Can you work these out from the model? Positions are in its coordinate system, mm. Face numbers are marked on the shaded views. A direction names the side the tool comes from. Give positions to 0.01 mm unless a question says otherwise; leave off trailing zeros. Order: outer loops, then holes, each group sorted by start corner. A loop starts at its lowest first (then second) coordinate and runs counter-clockwise, first axis right, second up. Notation, with made-up numbers: (21.5, 7.25) - (36.5, 7.25) arc R32 cw to (36.5, 41.25) - close; hole circle Ø5 at (18, 32). An arc over 180 degrees is marked (long way). Answer as CSV lines item,"result".
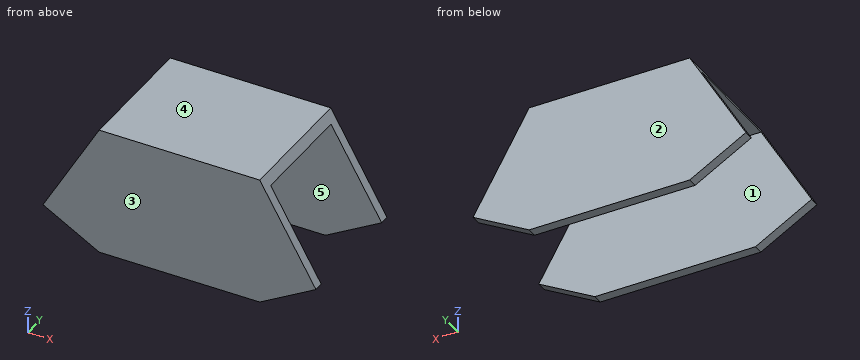
```python
from build123d import *

# Parameters (mm, degrees)
EXTRUDE_1_DEPTH = 40
SHELL_1_T       = -3


with BuildPart() as part:
    # 草图1 → 凸台-拉伸1 (new body)
    with BuildSketch(Plane(origin=(0, 0, 0), x_dir=(1, 0, 0), z_dir=(0, 1, 0))):
        Polygon((-25, -16.701458194), (25, -16.701458194), (42.5, 13.609430939), (25, 23.487817083), (-25, 23.487817083), (-42.5, 13.609430939), align=None)
    extrude(amount=EXTRUDE_1_DEPTH)

    # 抽壳1
    shell_1_openings = [part.faces().sort_by_distance(p)[0] for p in [
        (-33.75, 20, -18.548624011),
        (0, 20, -23.487817083),
        (33.75, 20, -18.548624011),
        (33.75, 20, 1.546013628),
        (-33.75, 20, 1.546013628),
    ]]
    offset(amount=SHELL_1_T, openings=shell_1_openings, kind=Kind.INTERSECTION)


solid = part.part
```
1) I want a section at C-C on x = 36.5. Write out the boundary of the cut face in (y, z).
Answer block:
outline,"(0, -17) - (3, -17) - (3, -3.22) - (0, -3.22) - close; (37, -17) - (40, -17) - (40, -3.22) - (37, -3.22) - close"
2) Which directions (+Z, -Z, +X, -X, +Y, -Y) give clear straight access to the entire face, cutting with the end or side of a thin tool? Please do the marked faces 4 and 5.
Answer block:
face 4,"+Z, +X, -X, +Y, -Y"
face 5,"-Z, +X, -X"
3) I want a section at A-A on z = 2.5. Write out the boundary of the cut face in (x, y).
Answer block:
outline,"(-33.2, 0) - (33.2, 0) - (33.2, 3) - (-33.2, 3) - close; (-33.2, 37) - (33.2, 37) - (33.2, 40) - (-33.2, 40) - close"
4) I need wall thicknesses on line 1 along Y through (x, z) = (-16.5, -15); line 2 along Z through (x, y) = (20, 28.5); line 3 along X through (y, z) = (38.5, 11). Which ranges of each line are inside material? Lowest first, please. Write a range as [from, to].
Answer block:
line 1,"[0, 3], [37, 40]"
line 2,"[13.7, 16.7]"
line 3,"[-28.29, 28.29]"
5) If we mould it in two halves opening along Y, with no side actions, what happens to the marked faces 1, 2 and 3? For each: +Y half, -Y half, draft (parallel to the pull), parting line (faces both ways), or undercut.
Answer block:
face 1,"undercut"
face 2,"+Y half"
face 3,"-Y half"
6) I'm going to push a flat-ended pin straight in: P1, Ø17, axis at x = -7.5, y = 12, coming from the -Z side. Where does the tip first touch, or does it pass through?
Answer block:
P1,"z = 13.7"
7) I want a section at B-B on x = -11.5. Write out the boundary of the cut face in (y, z), plus the area to 3 significant figures.
Answer block:
outline,"(0, -23.49) - (3, -23.49) - (3, 13.7) - (37, 13.7) - (37, -23.49) - (40, -23.49) - (40, 16.7) - (0, 16.7) - close"
area,"343 mm2"
8) I want a section at D-D on y = 22. Write out the boundary of the cut face in (x, z).
Answer block:
outline,"(-26.73, 13.7) - (26.73, 13.7) - (25, 16.7) - (-25, 16.7) - close"
